Autodesk Inventor part; units mm, degrees
ref_plane "YZ Plane" through (0, 0, 0) normal (1, 0, 0) x (0, 1, 0)
ref_plane "XZ Plane" through (0, 0, 0) normal (0, 1, 0) x (-1, 0, 0)
ref_plane "XY Plane" through (0, 0, 0) normal (0, 0, 1) x (1, 0, 0)
ref_plane "Arbeitsebene1" through (796.2209, 70.6141, -996.2958) normal (0, 0, -1) x (-1, 0, 0)
sketch "Skizze1" plane through (796.2209, 70.6141, -996.2958) normal (0, 0, -1) x (-1, 0, 0)
  line L0 (-3.9996, -76.75) -> (4.0004, -76.75) construction
  line L1 (-3.9996, 76.75) -> (-3.9996, -76.75) construction
  line L2 (4.0004, 76.75) -> (-3.9996, 76.75) construction
  line L3 (4.0004, 84.25) -> (4.0004, 76.75) construction
  line L4 (-37.8996, 84.25) -> (4.0004, 84.25) construction
  line L5 (-37.8996, 1.75) -> (-37.8996, 84.25) construction
  line L6 (-133.3996, 1.75) -> (-37.8996, 1.75) construction
  line L7 (-133.3996, -84.25) -> (-133.3996, 1.75) construction
  line L8 (4.0004, -84.25) -> (-133.3996, -84.25) construction
  line L9 (4.0004, -76.75) -> (4.0004, -84.25) construction
  line L10 (150.8004, -76.75) -> (142.8004, -76.75) construction
  line L11 (142.8004, -76.75) -> (142.8004, -84.25) construction
  line L12 (142.8004, -84.25) -> (280.2004, -84.25) construction
  line L13 (280.2004, -84.25) -> (280.2004, 1.75) construction
  line L14 (280.2004, 1.75) -> (184.7004, 1.75) construction
  line L15 (184.7004, 1.75) -> (184.7004, 84.25) construction
  line L16 (184.7004, 84.25) -> (142.8004, 84.25) construction
  line L17 (142.8004, 84.25) -> (142.8004, 76.75) construction
  line L18 (142.8004, 76.75) -> (150.8004, 76.75) construction
  line L19 (150.8004, 76.75) -> (150.8004, -76.75) construction
  line L20 (-5.9996, 76.75) -> (-5.9996, -76.75)
  line L21 (152.8004, 76.75) -> (152.8004, -76.75)
  line L22 (-5.9996, 76.75) -> (152.8004, 76.75)
  line L23 (-5.9996, -76.75) -> (152.8004, -76.75)
  point P0 (796.2209, -70.6141)
extrude "Extrusion1" add sketch "Skizze1" along normal blind 2
sketch "Skizze2" plane through (796.2209, 70.6141, -996.2958) normal (0, 0, 1) x (1, 0, 0)
  line L0 (-152.8004, -76.75) -> (-142.8004, -76.75)
  line L1 (-142.8004, -66.75) -> (-152.8004, -66.75)
  line L2 (-142.8004, -76.75) -> (-142.8004, -66.75)
  line L3 (-152.8004, -66.75) -> (-152.8004, -76.75)
  line L4 (-4.0004, -66.75) -> (5.9996, -66.75)
  line L5 (-4.0004, -76.75) -> (-4.0004, -66.75)
  line L6 (5.9996, -66.75) -> (5.9996, -76.75)
  line L7 (5.9996, -76.75) -> (-4.0004, -76.75)
  line L8 (-152.8004, 66.75) -> (-142.8004, 66.75)
  line L9 (-142.8004, 66.75) -> (-142.8004, 76.75)
  line L10 (-142.8004, 76.75) -> (-152.8004, 76.75)
  line L11 (-152.8004, 76.75) -> (-152.8004, 66.75)
  line L12 (-4.0004, 66.75) -> (-4.0004, 76.75)
  line L13 (5.9996, 66.75) -> (-4.0004, 66.75)
  line L14 (-4.0004, 76.75) -> (5.9996, 76.75)
  line L15 (5.9996, 76.75) -> (5.9996, 66.75)
  point P0 (-796.2209, -70.6141)
extrude "Extrusion2" add sketch "Skizze2" along normal blind 3.5
sketch "Skizze3" plane through (796.2209, 70.6141, -992.7958) normal (0, 0, 1) x (1, 0, 0)
  circle A0 centre (0.9996, 71.75) radius 1.75
  circle A1 centre (0.9996, -71.75) radius 1.75
  circle A2 centre (-147.8004, 71.75) radius 1.75
  circle A3 centre (-147.8004, -71.75) radius 1.75
  point P0 (-796.2209, -70.6141)
extrude "Extrusion3" cut sketch "Skizze3" against normal blind 15.5
sketch "Skizze4" plane through (796.2209, 70.6141, -998.2958) normal (0, 0, -1) x (-1, 0, 0)
  circle A0 centre (-0.9996, 71.75) radius 1.75
  circle A1 centre (-0.9996, 71.75) radius 3
  circle A2 centre (-0.9996, -71.75) radius 1.75
  circle A3 centre (147.8004, -71.75) radius 1.75
  circle A4 centre (147.8004, 71.75) radius 1.75
  circle A5 centre (147.8004, 71.75) radius 1.75
  circle A6 centre (147.8004, 71.75) radius 3
  circle A7 centre (-0.9996, -71.75) radius 1.75
  circle A8 centre (-0.9996, -71.75) radius 3
  circle A9 centre (147.8004, -71.75) radius 1.75
  circle A10 centre (147.8004, -71.75) radius 3
  point P0 (796.2209, -70.6141)
  dimension "d20" = 6
  dimension "d21" = 6
  dimension "d22" = 6
  dimension "d23" = 6
extrude "Extrusion4" cut sketch "Skizze4" against normal blind 3.4
equation "\"d21\" = d20"
equation "\"d22\" = d21"
equation "\"d23\" = d21"
properties part number "Backplate-housing"
Input: part model. Units: mm. Frame: model coordinates. A direction names the side the tool comes from. Coordinates: 2 decimals unless noted, no trailing zeros. Loops run counter-clockwise (first coordinate to the right, second up) from the corner with the lowest first, then second, coordinate; pieces in that order, holes last.
Q1. Cut plane B-B (y = 7). Output: boundary loops of the cut face in (x, z).
Q2. Draft query along X for faces 4 (the face through (647, 141, -994.896)), 5 (the face through (802.22, 72, -997)), 6 (the face through (797, 137.364, -995)). Return one class per face: +X half, -X half, draft (parallel to the pull), parting line (faces both ways), or undercut.
Q3. Cut plane C-C (x = 790). Output: boundary loops of the cut face in (y, z), then the cut area to 3 significant figures.
Q4. Cut plane A-A (z = -993.7). Output: boundary loops of the cut face in (x, y), then the cut area to 3 significant figures.
Q5. Set-up query: faces 1 (the face through (645.56, 143.27, -996.62)), 2 (the face through (792.22, -1, -995)), 3 (the face through (647.03, -2.2, -993.83)). Return all of +Z, -Z, +X, -X, +Y, -Y with unobstructed straight access to the full face (end or side cutting, diameter ignored); none if empty.
Q6. Material intervals for line 1 (Z direction, x = 666, y = 32.5); line 2 (X direction, y = 139, z = -995.5); line 3 (X direction, y = 141.5, z = -996.5), sorted ascending.
Q7. Contact query for flat-ended pins moving along their axis: pin 1 (5.5 mm diameter, centred on x = 648.42, y = 142.36, fed in from -Z); pin 2 (3 mm diameter, centred on x = 688.5, z = -994, fed in from -Y); pin 3 (2 mm diameter, centred on x = 672, y = 59, fed in from +Z). Output: stop coordinate, or through.
Working result:
1. outline: (643.42, -998.3) - (802.22, -998.3) - (802.22, -996.3) - (643.42, -996.3) - close
2. face 4: undercut
2. face 5: +X half
2. face 6: draft
3. outline: (-6.14, -998.3) - (147.36, -998.3) - (147.36, -996.3) - (-6.14, -996.3) - close
3. area: 307 mm2
4. outline: (643.42, -6.14) - (653.42, -6.14) - (653.42, 3.86) - (643.42, 3.86) - close; (643.42, 137.36) - (653.42, 137.36) - (653.42, 147.36) - (643.42, 147.36) - close; (792.22, -6.14) - (802.22, -6.14) - (802.22, 3.86) - (792.22, 3.86) - close; (792.22, 137.36) - (802.22, 137.36) - (802.22, 147.36) - (792.22, 147.36) - close; hole circle Ø3.5 at (648.42, -1.14); hole circle Ø3.5 at (648.42, 142.36); hole circle Ø3.5 at (797.22, -1.14); hole circle Ø3.5 at (797.22, 142.36)
4. area: 362 mm2
5. face 1: -Z
5. face 2: +Z, +Y, -Y
5. face 3: +Z, -Z
6. line 1: z = -998.3 to -996.3
6. line 2: x = 643.42 to 653.42, 792.22 to 802.22
6. line 3: x = 643.42 to 645.55, 651.29 to 794.35, 800.09 to 802.22
7. pin 1: stops at z = -994.9
7. pin 2: passes through
7. pin 3: stops at z = -996.3
